For this review, take the finished solid that the model builds, in its own axes (mm). Face numbers are marked on the shaded views. A direction names the side the tool comes from. Round coordinates to 2 decimals unless told otherwise and drop trailing zeros. Loops run counter-clockwise (first coordinate to the right, second up) from the corner with the lowest first, then second, coordinate; pieces in that order, holes last.
1) Take a section at B-B (z = 4.5). State the section outline as (x, y) points, then the cut area to 3 significant figures.
2) Take a section at A-A (x = 25). State the section outline as (y, z) points, then the cut area to 3 significant figures.
3) Take a section at C-C (y = 6). State the section outline as (x, z) points.
4) Tool access review of the marked faces 4 and 5: name each direction out of +Z, -Z, +X, -X, +Y, -Y from which nothing blocks a thin tool from reaching the whole face with its end or side.
5) Take a section at D-D (z = 7). State the section outline as (x, y) points.
6) Wall thickness on L1, parallel to Y at x = 25, z = 11.2; L2, parallel to Y at x = 25, z = 4.25; L3, parallel to Y at x = 18, z = 3.25: over which ranges is each line inside the solid? List them lowest first.
7) Insertion check: pin 1 (5 mm diameter, centred on x = 20, z = 5.5, fed in from -Y); pin 2 (6 mm diameter, centred on x = 37, z = 10.5, fed in from +Y); pin 3 (7 mm diameter, centred on x = 4.97, z = 6, fed in from -Y). Each pin has a flat end and moves straight along its axis. Give the tip position at first contact, or say it passes through.
8) Mouldability with a two-part tool opening along Z and no side actions: class the marked faces 1, 2 and 3 as pulls with the +Z half, pulls with the -Z half, needs draft (parallel to the pull), parting line crosses it, or undercut.
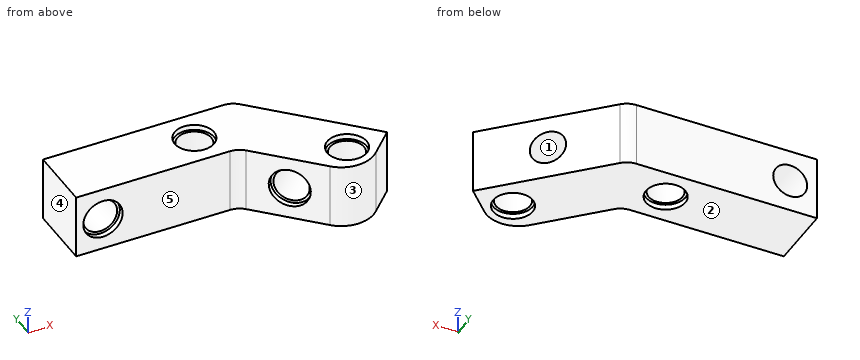
```python
from build123d import *

# Parameters (mm, degrees)
BOSS_EXTRU_1_DEPTH           = 12
ESQUISSE2_R                  = 3.15
ENL_V_MAT_EXTRU_1_DEPTH      = 1
ENL_V_MAT_EXTRU_1_DEPTH_BACK = 13
ESQUISSE3_R                  = 3.15
ENL_V_MAT_EXTRU_2_DEPTH      = 12
ESQUISSE4_R                  = 3.15
ENL_V_MAT_EXTRU_3_DEPTH      = 1
ENL_V_MAT_EXTRU_3_DEPTH_BACK = 28.556349186
ESQUISSE5_R                  = 3.65
ENL_V_MAT_EXTRU_4_DEPTH      = 1
ESQUISSE6_R                  = 3.65
ENL_V_MAT_EXTRU_5_DEPTH      = 1
ESQUISSE7_R                  = 3.65
ENL_V_MAT_EXTRU_6_DEPTH      = 1
ESQUISSE8_R                  = 3.65
ENL_V_MAT_EXTRU_7_DEPTH      = 1
CONG_1_R                     = 3.5
CONG_2_R                     = 6


with BuildPart() as part:
    # Esquisse1 → Boss.-Extru.1 (new body)
    with BuildSketch(Plane.XY):
        Polygon((0, 0), (30, 0), (45.556349186, -15.556349186), (54.04163056, -7.071067812), (34.970562748, 12), (0, 12), align=None)
    extrude(amount=BOSS_EXTRU_1_DEPTH)

    # Esquisse2 → Enlèv. mat.-Extru.1 (cut, two sides)
    with BuildSketch(Plane.XY.offset(12)) as enl_v_mat_extru_1_sk:
        with Locations((25, 6)):
            Circle(ESQUISSE2_R)
        with Locations((46.263455967, -7.778174593)):
            Circle(ESQUISSE2_R)
    extrude(amount=ENL_V_MAT_EXTRU_1_DEPTH, mode=Mode.SUBTRACT)
    extrude(enl_v_mat_extru_1_sk.sketch, amount=-ENL_V_MAT_EXTRU_1_DEPTH_BACK, mode=Mode.SUBTRACT)

    # Esquisse3 → Enlèv. mat.-Extru.2 (cut)
    with BuildSketch(Plane(origin=(23.485281374, 23.485281374, 0), x_dir=(0, 0, -1), z_dir=(0.707106781, 0.707106781, 0))):
        with Locations((-6, -30.213203436)):
            Circle(ESQUISSE3_R)
    extrude(amount=-ENL_V_MAT_EXTRU_2_DEPTH, mode=Mode.SUBTRACT)

    # Esquisse4 → Enlèv. mat.-Extru.3 (cut, two sides)
    with BuildSketch(Plane(origin=(0, 12, 0), x_dir=(1, 0, 0), z_dir=(0, 1, 0))) as enl_v_mat_extru_3_sk:
        with Locations((4.970562748, -6)):
            Circle(ESQUISSE4_R)
    extrude(amount=ENL_V_MAT_EXTRU_3_DEPTH, mode=Mode.SUBTRACT)
    extrude(enl_v_mat_extru_3_sk.sketch, amount=-ENL_V_MAT_EXTRU_3_DEPTH_BACK, mode=Mode.SUBTRACT)

    # Esquisse5 → Enlèv. mat.-Extru.4 (cut)
    with BuildSketch(Plane.XY.offset(12)):
        with Locations((25, 6)):
            Circle(ESQUISSE5_R)
        with Locations((46.263455967, -7.778174593)):
            Circle(ESQUISSE5_R)
    extrude(amount=-ENL_V_MAT_EXTRU_4_DEPTH, mode=Mode.SUBTRACT)

    # Esquisse6 → Enlèv. mat.-Extru.5 (cut)
    with BuildSketch(Plane(origin=(0, 0, 0), x_dir=(-1, 0, 0), z_dir=(0, 0, -1))):
        with Locations((-25, 6)):
            Circle(ESQUISSE6_R)
        with Locations((-46.263455967, -7.778174593)):
            Circle(ESQUISSE6_R)
    extrude(amount=-ENL_V_MAT_EXTRU_5_DEPTH, mode=Mode.SUBTRACT)

    # Esquisse7 → Enlèv. mat.-Extru.6 (cut)
    with BuildSketch(Plane(origin=(15, 15, 0), x_dir=(0, 0, 1), z_dir=(-0.707106781, -0.707106781, 0))):
        with Locations((6, -30.213203436)):
            Circle(ESQUISSE7_R)
    extrude(amount=-ENL_V_MAT_EXTRU_6_DEPTH, mode=Mode.SUBTRACT)

    # Esquisse8 → Enlèv. mat.-Extru.7 (cut)
    with BuildSketch(Plane.XZ):
        with Locations((4.970562748, 6)):
            Circle(ESQUISSE8_R)
    extrude(amount=-ENL_V_MAT_EXTRU_7_DEPTH, mode=Mode.SUBTRACT)

    # Congé1
    cong_1_edges = [part.edges().sort_by_distance(p)[0] for p in [
        (34.970562748, 12, 6),
        (30, 0, 6),
    ]]
    fillet(cong_1_edges, radius=CONG_1_R)

    # Congé2
    cong_2_edges = [part.edges().sort_by_distance(p)[0] for p in [
        (45.556349186, -15.556349186, 6),
    ]]
    fillet(cong_2_edges, radius=CONG_2_R)


solid = part.part
```
Response:
1. outline: (0, 0) - (1.64, 0) - (1.64, 1) - (2.2, 1) - (2.2, 12) - (0, 12) - close; (7.74, 1) - (8.3, 1) - (8.3, 0) - (28.55, 0) arc R3.5 cw to (31.03, -1.03) - (34.01, -4.01) - (34.72, -3.3) - (35.11, -3.7) - (42.89, 4.08) - (36, 10.97) arc R3.5 ccw to (33.52, 12) - (7.74, 12) - close; (38.72, -8.72) - (41.31, -11.31) arc R6 ccw to (49.8, -11.31) - (54.04, -7.07) - (46.81, 0.16) - (39.03, -7.62) - (39.42, -8.01) - close; hole circle Ø6.3 at (25, 6); hole circle Ø6.3 at (46.26, -7.78)
1. area: 478 mm2
2. outline: (0, 0) - (2.35, 0) - (2.35, 1) - (2.85, 1) - (2.85, 11) - (2.35, 11) - (2.35, 12) - (0, 12) - close; (9.15, 1) - (9.65, 1) - (9.65, 0) - (12, 0) - (12, 12) - (9.65, 12) - (9.65, 11) - (9.15, 11) - close
2. area: 66.4 mm2
3. outline: (0, 0) - (21.35, 0) - (21.35, 1) - (21.85, 1) - (21.85, 11) - (21.35, 11) - (21.35, 12) - (0, 12) - close; (28.15, 1) - (28.65, 1) - (28.65, 0) - (40.97, 0) - (40.97, 12) - (28.65, 12) - (28.65, 11) - (28.15, 11) - close; hole circle Ø6.3 at (4.97, 6)
4. face 4: +Z, -Z, -X, +Y, -Y
4. face 5: +Z, -Z, -X, -Y
5. outline: (0, 0) - (1.46, 0) - (1.46, 1) - (1.98, 1) - (1.98, 12) - (0, 12) - close; (7.96, 1) - (8.48, 1) - (8.48, 0) - (28.55, 0) arc R3.5 cw to (31.03, -1.03) - (33.88, -3.88) - (34.59, -3.17) - (34.96, -3.54) - (42.74, 4.23) - (36, 10.97) arc R3.5 ccw to (33.52, 12) - (7.96, 12) - close; (38.85, -8.85) - (41.31, -11.31) arc R6 ccw to (49.8, -11.31) - (54.04, -7.07) - (46.96, 0.01) - (39.18, -7.77) - (39.55, -8.14) - close; hole circle Ø6.3 at (25, 6); hole circle Ø6.3 at (46.26, -7.78)
6. L1: y = 0 to 2.35, 9.65 to 12
6. L2: y = 0 to 2.85, 9.15 to 12
6. L3: y = 0 to 12
7. pin 1: stops at y = 0
7. pin 2: stops at y = 11.97
7. pin 3: stops at y = 1
8. face 1: undercut
8. face 2: pulls with the -Z half
8. face 3: needs draft
